from build123d import *

# Parameters (mm, degrees)
AUFSATZ_LINEAR_AUSTRAGEN1_DEPTH = 2


with BuildPart() as part:
    # Skizze1 → Aufsatz-Linear austragen1 (new body)
    with BuildSketch(Plane.XY):
        with BuildLine():
            Line((-49.2275, -51.8905), (-49.2275, -151.2967))
            ThreePointArc((-49.2275, -151.2967), (-52.244300154, -158.579899846), (-59.5275, -161.5967))
            Line((-59.5275, -161.5967), (-169.0581, -161.5967))
            ThreePointArc((-169.0581, -161.5967), (-176.514004305, -158.403485592), (-179.34742314, -150.803560266))
            Line((-179.34742314, -150.803560266), (-179.34742314, -52.3842))
            ThreePointArc((-179.34742314, -52.3842), (-176.514207067, -44.783915623), (-169.0581, -41.5905))
            Line((-169.0581, -41.5905), (-59.5275, -41.5905))
            ThreePointArc((-59.5275, -41.5905), (-52.244300154, -44.607300154), (-49.2275, -51.8905))
        make_face()
        with BuildLine():
            Line((-59.5275, -152.0967), (-169.0581, -152.0967))
            ThreePointArc((-169.0581, -152.0967), (-169.972884043, -151.717784043), (-170.3518, -150.803))
            Line((-170.3518, -150.803), (-170.3518, -52.3842))
            ThreePointArc((-170.3518, -52.3842), (-169.972884043, -51.469415957), (-169.0581, -51.0905))
            Line((-169.0581, -51.0905), (-59.5275, -51.0905))
            ThreePointArc((-59.5275, -51.0905), (-58.612715957, -51.469415957), (-58.2338, -52.3842))
            Line((-58.2338, -52.3842), (-58.2338, -150.803))
            ThreePointArc((-58.2338, -150.803), (-58.612715957, -151.717784043), (-59.5275, -152.0967))
        make_face(mode=Mode.SUBTRACT)
        Polygon((-57.8838, -155.0967), (-56.659055129, -152.7467), (-53.808544871, -152.7467), (-52.5838, -155.0967), (-53.808544871, -157.4467), (-56.659055129, -157.4467), align=None, mode=Mode.SUBTRACT)
        Polygon((-171.422168012, -157.4467), (-170.19742314, -155.0967), (-171.422168012, -152.7467), (-174.272678269, -152.7467), (-175.49742314, -155.0967), (-174.272678269, -157.4467), align=None, mode=Mode.SUBTRACT)
        Polygon((-175.49742314, -48.0905), (-174.272678269, -45.7405), (-171.422168012, -45.7405), (-170.19742314, -48.0905), (-171.422168012, -50.4405), (-174.272678269, -50.4405), align=None, mode=Mode.SUBTRACT)
        Polygon((-57.8838, -48.0905), (-56.659055129, -45.7405), (-53.808544871, -45.7405), (-52.5838, -48.0905), (-53.808544871, -50.4405), (-56.659055129, -50.4405), align=None, mode=Mode.SUBTRACT)
    extrude(amount=AUFSATZ_LINEAR_AUSTRAGEN1_DEPTH)


solid = part.part
The listing builds one solid part. Answer for the finished solid, in the listing's coordinates (mm). Give positions to 0.01 mm unless a question says otherwise; leave off trailing zeros. Order: outer loops, then holes, each group sorted by start corner. A loop starts at its lowest first (then second) coordinate and runs counter-clockwise, first axis right, second up. Notation, with made-up numbers: (62, 69) - (76, 69) arc R20 cw to (76, 81) - close; hole circle Ø6 at (51.25, 5.25). An arc over 180 degrees is marked (long way). Use one line per item in the form item = value.
1) Consider probe 1 along Y at (x, z) = (-157, 0.5); probe 2 along X at (y, z) = (-87, 0.65); probe 3 along X at (y, z) = (-154, 1.65). Determine where each line is inside the solid, lowest interval first. Write a range as [from, to].
Verdict:
probe_1 = [-161.6, -152.1], [-51.09, -41.59]
probe_2 = [-179.35, -170.35], [-58.23, -49.23]
probe_3 = [-179, -174.93], [-170.77, -57.31], [-53.16, -49.59]
2) Find section C-C on z = 0.5. Give the number of separate pieces and of enclosed holes in the cut face, and give its area (3 significant figures).
Verdict:
separate_pieces = 1
enclosed_holes = 5
area = 4,120 mm^2
3) Find section B-B on x = -101. Determine the outline of the cut face in (y, z).
Verdict:
outline = (-161.6, 0) - (-152.1, 0) - (-152.1, 2) - (-161.6, 2) - close; (-51.09, 0) - (-41.59, 0) - (-41.59, 2) - (-51.09, 2) - close
4) Each of these flat-tipped pins is pushed along its axis until it touches: pin 1 (1 mm diameter, centred on x = -55, z = 0.5, fed in from +Y); pin 2 (0.6 mm diameter, centred on x = -172.5, z = 1, fed in from -Y); pin 3 (0.6 mm diameter, centred on x = -173.5, z = 0.5, fed in from +Y); pin 4 (5 mm diameter, centred on x = -91, y = -148, fed in from -Z). Where does it stop, or does it pass through?
Verdict:
pin_1 = -42.41
pin_2 = -161.11
pin_3 = -42.46
pin_4 = through
5) Find section A-A on y = -75. Determine the outline of the cut face in (x, z).
Verdict:
outline = (-179.35, 0) - (-170.35, 0) - (-170.35, 2) - (-179.35, 2) - close; (-58.23, 0) - (-49.23, 0) - (-49.23, 2) - (-58.23, 2) - close
